from build123d import *

# Parameters (mm, degrees)
SKETCH1_W           = 276
SKETCH1_H           = 300
BOSS_EXTRUDE1_DEPTH = 1.5
SKETCH2_W           = 1.5
SKETCH2_H           = 300
BOSS_EXTRUDE2_DEPTH = 20
FILLET1_R           = 1


with BuildPart() as part:
    # Sketch1 → Boss-Extrude1 (new body)
    with BuildSketch(Plane(origin=(0, 0, 0), x_dir=(1, 0, 0), z_dir=(0, 1, 0))):
        Rectangle(SKETCH1_W, SKETCH1_H)
    extrude(amount=BOSS_EXTRUDE1_DEPTH)

    # Sketch2 → Boss-Extrude2 (add)
    with BuildSketch(Plane(origin=(0, 1.5, 0), x_dir=(1, 0, 0), z_dir=(0, 1, 0))):
        with Locations((-137.25, 0)):
            Rectangle(SKETCH2_W, SKETCH2_H)
        with Locations((137.25, 0)):
            Rectangle(SKETCH2_W, SKETCH2_H)
    extrude(amount=BOSS_EXTRUDE2_DEPTH)

    # Fillet1
    fillet1_edges = [part.edges().sort_by_distance(p)[0] for p in [
        (-138, 0, 0),
        (138, 0, 0),
    ]]
    fillet(fillet1_edges, radius=FILLET1_R)


solid = part.part
Verification items for the finished model (mm, model axes). A direction names the side the tool comes from. Coordinates: 2 decimals unless noted, no trailing zeros. Loops run counter-clockwise (first coordinate to the right, second up) from the corner with the lowest first, then second, coordinate; pieces in that order, holes last. Notation, with made-up numbers: (-18.75, 85.5) -> (-8.75, 85.5) arc R14 cw to (-8.75, 109.5) -> close; hole circle Ø4 at (41.5, 4). An arc over 180 degrees is marked (long way). Write each question's results on one line, items separated by ' | '.
Item 1: Section check C-C, the plane x = 67.5. Enter the section's corners in (y, z).
Found:
outline: (0, -150) -> (1.5, -150) -> (1.5, 150) -> (0, 150) -> close
Item 2: Mould release check, pull along X, two halves, no side actions. Record for faces 3 (the face through (138, 11, 2)), 4 (the face through (-136.5, 11, 2)), 5 (the face through (-0.6, 0.3, -150)): +X half, -X half, draft (parallel to the pull), parting line (faces both ways), or undercut.
Found:
face 3: +X half | face 4: undercut | face 5: draft
Item 3: Gauge pin test, flat end, axial feed: pin 1 (6 mm diameter, centred on x = 55, z = 47.5, fed in from +Y). Record the tip position at first contact, or that the pin passes through.
Found:
pin 1: stops at y = 1.5
Item 4: Section check B-B, the plane z = -125. Enter the section's corners in (x, y), plus the area to 3 significant figures.
Found:
outline: (-138, 1) arc R1 ccw to (-137, 0) -> (137, 0) arc R1 ccw to (138, 1) -> (138, 21.5) -> (136.5, 21.5) -> (136.5, 1.5) -> (-136.5, 1.5) -> (-136.5, 21.5) -> (-138, 21.5) -> close | area: 474 mm2
Item 5: Tool access check on faces 1 (the face through (-138, 11, 2)), 2 (the face through (-2, 1.5, -2)). Record the directions out of +Z, -Z, +X, -X, +Y, -Y that give a thin tool (end or side, any length) a straight path to the whole face; none if there is none.
Found:
face 1: +Z, -Z, -X, +Y, -Y | face 2: +Z, -Z, +Y
Item 6: Material ranges on L1, parallel to X at y = 2.5, z = 103; L2, parallel to Y at x = 19, z = -112, recorded low to high.
Found:
L1: x = -138 to -136.5, 136.5 to 138 | L2: y = 0 to 1.5
Item 7: Section check A-A, the plane y = 18.25. Enter the section's corners in (x, z), plus the area to 3 significant figures.
Found:
outline: (-138, -150) -> (-136.5, -150) -> (-136.5, 150) -> (-138, 150) -> close; (136.5, -150) -> (138, -150) -> (138, 150) -> (136.5, 150) -> close | area: 900 mm2
